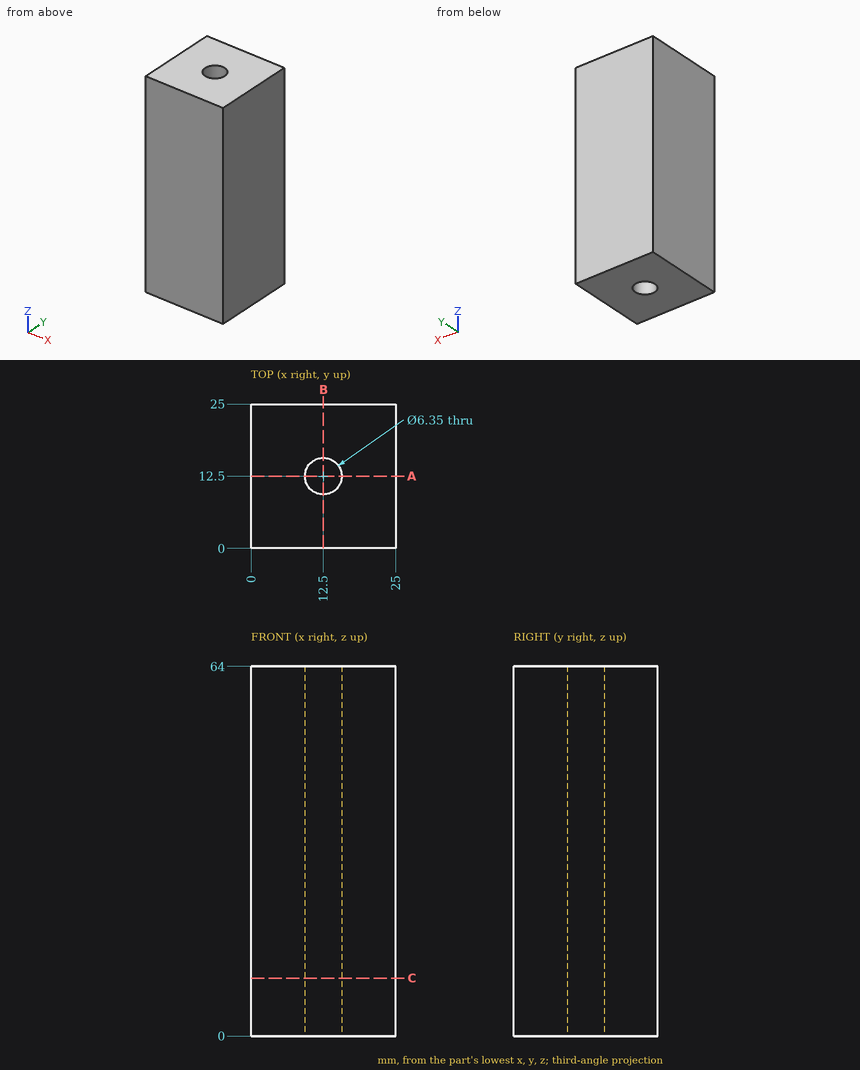
Input: dimensioned drawing with shaded views. Units: mm. Origin: part minimum x, y, z. Round coordinates to 2 decimals unless told otherwise and drop trailing zeros. Order: outer loops, then holes, each group sorted by start corner. A loop starts at its lowest first (then second) coordinate and runs counter-clockwise, first axis right, second up. Notation, with made-up numbers: (82.25, 67.5) - (133.25, 67.5) arc R14 ccw to (133.25, 93.5) - close; hole circle Ø6 at (14.25, 10). An arc over 180 degrees is marked (long way). Answer as a JSON object with one key per item and string values. Group by question number.
(1) Cut plane A-A (y = 12.5). Return loops of the section in (x, z) (3 decimals).
(2) Cut plane C-C (z = 10). Return loops of the section in (x, y) (3 decimals).
(3) Material intervals for probe 1 along X at (y, z) = (12.5, 39.5) (3 decimals); probe 2 along X at (y, z) = (13.75, 16.5); probe 3 along Y at (x, z) = (15.25, 17), sorted ascending. Write a range as from..to.
Here are the results:
{
 "1": {"outline": "(0, 0) - (9.325, 0) - (9.325, 64) - (0, 64) - close; (15.675, 0) - (25, 0) - (25, 64) - (15.675, 64) - close"},
 "2": {"outline": "(0, 0) - (25, 0) - (25, 25) - (0, 25) - close; hole circle Ø6.35 at (12.5, 12.5)"},
 "3": {"probe 1": "x = 0..9.325, 15.675..25", "probe 2": "x = 0..9.58, 15.42..25", "probe 3": "y = 0..10.91, 14.09..25"}
}
